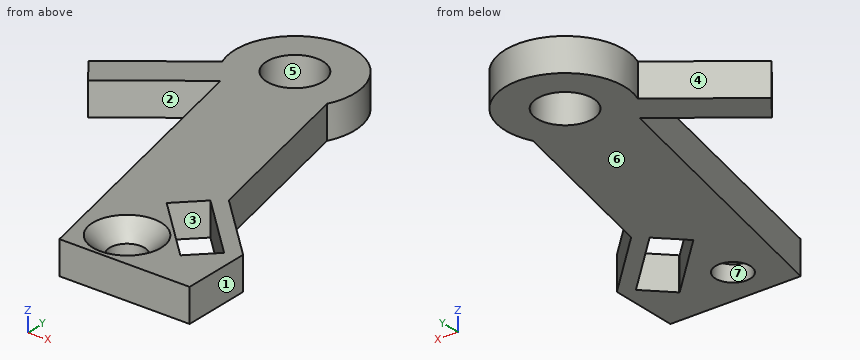
```python
from build123d import *

# Parameters (mm, degrees)
SKETCH1_R           = 1.5
SKETCH1_R_2         = 2.575
BOSS_EXTRUDE1_DEPTH = 3.05


with BuildPart() as part:
    # Sketch1 → Boss-Extrude1 (new body)
    with BuildSketch(Plane.XY):
        with BuildLine():
            Line((5.98959236, 12.314316255), (2.43581293, 28.4362191))
            ThreePointArc((2.43581293, 28.4362191), (-2.208633676, 36.424535456), (-7.57966444, 28.905485582))
            Line((-7.57966444, 28.905485582), (-15.289043869, 23.004605125))
            Line((-15.289043869, 23.004605125), (-13.465626641, 20.622347873))
            Line((-13.465626641, 20.622347873), (-5.833523684, 26.464079701))
            Line((-5.833523684, 26.464079701), (0, 0))
            Line((0, 0), (12, 0))
            Line((12, 0), (12, 6.303908615))
            Line((12, 6.303908615), (5.98959236, 12.314316255))
        make_face()
        with Locations((3.5, 3.5)):
            Circle(SKETCH1_R, mode=Mode.SUBTRACT)
        Polygon((10.727207794, 5.692209589), (8.517499103, 3.482500897), (8.464466094, 3.429467889), (2.701545827, 9.192388155), (4.964287527, 11.455129855), align=None, mode=Mode.SUBTRACT)
        with Locations((-2.466048994, 30.930562636)):
            Circle(SKETCH1_R_2, mode=Mode.SUBTRACT)
    extrude(amount=BOSS_EXTRUDE1_DEPTH)

    # Sketch3 → CSK for M3 Flat Head Machine Screw1 (revolve, cut)
    with BuildSketch(Plane(origin=(3.5, 3.5, 3.05), x_dir=(0, -1, 0), z_dir=(1, 0, 0))):
        Polygon((0, 0), (0, 3.05), (1.6, 3.05), (1.6, 1.55), (3.15, 0), align=None)
    revolve(axis=Axis((3.5, 3.5, 9.4), (0, 0, -1)), mode=Mode.SUBTRACT)


solid = part.part
```
Geometry check sheet. Reference: the model listing, model coordinates, mm. Face numbers are marked on the shaded views. A direction names the side the tool comes from. Give positions to 0.01 mm unless a question says otherwise; leave off trailing zeros. Order: outer loops, then holes, each group sorted by start corner. A loop starts at its lowest first (then second) coordinate and runs counter-clockwise, first axis right, second up. Notation, with made-up numbers: (10, -28) - (15, -28) arc R20 cw to (15, -6) - close; hole circle Ø3 at (68.25, 75). An arc over 180 degrees is marked (long way). Answer in a Markdown table with one row per item. Add a question column.
Q1. Tool access check on the marked faces 1, 2 and 3. Record the directions out of +Z, -Z, +X, -X, +Y, -Y that give a thin tool (end or side, any length) a straight path to the whole face; none if there is none.
Q2. Mould release check, pull along X, two halves, no side actions. Record for the marked faces 4, 5, 6 and 7: pulls with the +X half, pulls with the -X half, needs draft (parallel to the pull), parting line crosses it, or undercut.
Q3. Cross-section at D-D, the plane x = 10. Enter the section's corners in (y, z) (3 decimals), then the cut area to 3 significant figures.
Q4. Material ranges on probe 1 along Y at (x, z) = (10.5, 2.45) (3 decimals); probe 2 along Y at (x, z) = (7.75, 1.55); probe 3 along X at (y, z) = (25, 2.05), recorded low to high. Write a range as from..to.
Q5. Cross-section at B-B, the plane x = 3.5. Enter the section's corners in (y, z), then the cut area to 3 significant figures.
Q6. Gauge pin test, flat ends, axial feed: pin 1 (4.5 mm diameter, centred on x = -2.47, y = 30.93, fed in from -Z); pin 2 (4 mm diameter, centred on x = 3.5, y = 3.5, fed in from +Z); pin 3 (1.5 mm diameter, centred on y = 32.5, z = 2.5, fed in from -X). Record the tip position at first contact, or that the pin passes through.
Q7. Cross-section at A-A, the plane y = 33. Enter the section's corners in (x, z).
Q8. Cross-section at C-C, the plane z = 0.75. Count the separate pieces of the cut face and the enclosed holes in it, then the cut area to 3 significant figures.
Check values:
| question | item | result |
|---|---|---|
| 1 | face 1 | +Z, -Z, +X, +Y, -Y |
| 1 | face 2 | +Z, -Z, -Y |
| 1 | face 3 | +Z, -Z |
| 2 | face 4 | pulls with the -X half |
| 2 | face 5 | undercut |
| 2 | face 6 | needs draft |
| 2 | face 7 | undercut |
| 3 | outline | (0, 0) - (4.965, 0) - (4.965, 3.05) - (0, 3.05) - close; (6.419, 0) - (8.304, 0) - (8.304, 3.05) - (6.419, 3.05) - close |
| 3 | area | 20.9 mm^2 |
| 4 | probe 1 | y = 0..5.465, 5.919..7.804 |
| 4 | probe 2 | y = 0..4.14, 8.67..10.55 |
| 4 | probe 3 | x = -12.68..-7.75, -5.51..3.19 |
| 5 | outline | (0, 0) - (1.9, 0) - (1.9, 1.5) - (0.35, 3.05) - (0, 3.05) - close; (5.1, 0) - (8.39, 0) - (8.39, 3.05) - (6.65, 3.05) - (5.1, 1.5) - close; (9.99, 0) - (23.61, 0) - (23.61, 3.05) - (9.99, 3.05) - close |
| 5 | area | 55.0 mm^2 |
| 6 | pin 1 | passes through |
| 6 | pin 2 | stops at z = 1.9 |
| 6 | pin 3 | stops at x = -7.9 |
| 7 | outline | (-7.56, 0) - (-4, 0) - (-4, 3.05) - (-7.56, 3.05) - close; (-0.93, 0) - (2.63, 0) - (2.63, 3.05) - (-0.93, 3.05) - close |
| 8 | separate pieces | 1 |
| 8 | enclosed holes | 3 |
| 8 | area | 336 mm^2 |
